```python
from build123d import *
from build123d.topology import SkipClean

# Parameters (mm, degrees)
SKETCH1_3_W             = 80
SKETCH1_3_H             = 80
SKETCH1_3_R             = 15
SKETCH1_3_R_2           = 2.5
BOSS_EXTRUDE3_DEPTH     = 5
BOSS_EXTRUDE4_START     = 5
SKETCH1_W               = 80
SKETCH1_H               = 80
SKETCH1_R               = 2.5
SKETCH1_R_2             = 25
BOSS_EXTRUDE4_DEPTH     = 5
CUT_EXTRUDE2_DEPTH      = 57.789083458
CUT_EXTRUDE2_DEPTH_BACK = 57.789083458
CUT_EXTRUDE3_DEPTH      = 57.789083608
CUT_EXTRUDE3_DEPTH_BACK = 57.789083608


with BuildPart() as part:
    # Sketch1_3 → Boss-Extrude3 (new body)
    with BuildSketch(Plane(origin=(0, 0, 0), x_dir=(1, 0, 0), z_dir=(0, 1, 0))):
        Rectangle(SKETCH1_3_W, SKETCH1_3_H)
        with Locations(Location((0, 0, 0), (0, 0, 270))):
            Circle(SKETCH1_3_R, mode=Mode.SUBTRACT)
        with Locations(Location((-32, 32, 0), (0, 0, 270))):
            Circle(SKETCH1_3_R_2, mode=Mode.SUBTRACT)
        with Locations(Location((-32, -32, 0), (0, 0, 270))):
            Circle(SKETCH1_3_R_2, mode=Mode.SUBTRACT)
        with Locations(Location((32, -32, 0), (0, 0, 270))):
            Circle(SKETCH1_3_R_2, mode=Mode.SUBTRACT)
        with Locations(Location((32, 32, 0), (0, 0, 270))):
            Circle(SKETCH1_3_R_2, mode=Mode.SUBTRACT)
    extrude(amount=-BOSS_EXTRUDE3_DEPTH)

    # Sketch1 → Boss-Extrude4 (add)
    with BuildSketch(Plane(origin=(0, 0, 0), x_dir=(1, 0, 0), z_dir=(0, 1, 0)).offset(BOSS_EXTRUDE4_START)):
        Rectangle(SKETCH1_W, SKETCH1_H)
        with Locations(Location((-32, -32, 0), (0, 0, 270))):
            Circle(SKETCH1_R, mode=Mode.SUBTRACT)
        with Locations(Location((32, -32, 0), (0, 0, 270))):
            Circle(SKETCH1_R, mode=Mode.SUBTRACT)
        with Locations(Location((0, 0, 0), (0, 0, 270))):
            Circle(SKETCH1_R_2, mode=Mode.SUBTRACT)
        with Locations(Location((-32, 32, 0), (0, 0, 270))):
            Circle(SKETCH1_R, mode=Mode.SUBTRACT)
        with Locations(Location((32, 32, 0), (0, 0, 270))):
            Circle(SKETCH1_R, mode=Mode.SUBTRACT)
    extrude(amount=-BOSS_EXTRUDE4_DEPTH)

    # Sketch3 → Cut-Extrude2 (cut, two sides: drawn at the far end of the back side and taken through both)
    with BuildSketch(Plane.XY.offset(-CUT_EXTRUDE2_DEPTH_BACK)):
        with BuildLine():
            Line((-40, 1.643191324), (-40, 5))
            Line((-40, 5), (0, 5))
            ThreePointArc((0, 5), (-20.070302467, 4.159325469), (-40, 1.643191324))
        make_face()
    extrude(amount=CUT_EXTRUDE2_DEPTH + CUT_EXTRUDE2_DEPTH_BACK, mode=Mode.SUBTRACT)

    # Sketch3_4 → Cut-Extrude3 (cut, two sides: drawn at the far end of the back side and taken through both)
    with SkipClean():  # the faces are left unmerged after this step: merging them gives an invalid solid
        with BuildSketch(Plane.XY.offset(-CUT_EXTRUDE3_DEPTH_BACK)):
            with BuildLine():
                Line((40, 5), (40, 1.643191324))
                ThreePointArc((40, 1.643191324), (20.070302467, 4.159325469), (0, 5))
                Line((0, 5), (40, 5))
            make_face()
        extrude(amount=CUT_EXTRUDE3_DEPTH + CUT_EXTRUDE3_DEPTH_BACK, mode=Mode.SUBTRACT)


solid = part.part
```
Verification items for the finished model (mm, model axes). A direction names the side the tool comes from. Coordinates: 2 decimals unless noted, no trailing zeros. Write each loop counter-clockwise with the first axis right and the second up, starting at its lowest first coordinate (ties: lowest second). Pieces come first, ordered by that corner, then holes. Notation, with made-up numbers: (-30, 41) - (15, 41) arc R20 ccw to (15, 47) - close; hole circle Ø10 at (-6, 87). An arc over 180 degrees is marked (long way). One line per question, with ' | ' between items. Start each with the question number.
1. Material ranges on line 1 along X through (y, z) = (-2.25, -32); line 2 along X through (y, z) = (0, -34); line 3 along Z through (x, y) = (0, 4), recorded low to high.
2. Section check B-B (z = 0). Enter the section's corners in (x, y), plus the area to 3 significant figures.
3. Section check C-C (y = -3.5). Enter the section's corners in (x, z), plus the area to 3 significant figures.
4. Access from +Z, -Z, +X, -X, +Y, -Y to the whole of each face (thin tool, end or side, straight path). Record for faces 1 (the cylindrical face through (7.509, 1.979, 23.846)), 2 (the flat face through (40, -2, 1)).
5. Draft check along X on faces 3 (the flat face through (-1, 0, 40)), 4 (the cylindrical face through (-29.52, -0.85, -32.33)), 5 (the flat face through (-40, -2, 1)). Enter one of: released by +X, released by -X, zero draft, split by the parting line, or undercut.
6. Section check A-A (x = 32). Enter the section's corners in (y, z).
7. Gauge pin test, flat ends, axial feed: P1, Ø8, axis at x = 11, z = 3.5, coming from the +Y side; P2, Ø6.5, axis at x = -32, z = 32, coming from the -Y side; P3, Ø8, axis at x = -32, z = -32, coming from the +Y side; P4, Ø6.5, axis at x = 32, z = -32, coming from the +Y side. Record the tip position at first contact, or that the pin passes through.
8. Section check D-D (x = 7). Enter the section's corners in (y, z), plus the area to 3 significant figures.
Computed values:
1) line 1: -40 to -34.5, -29.5 to 29.5, 34.5 to 40 | line 2: -40 to -33.5, -30.5 to 30.5, 33.5 to 40 | line 3: -40 to -25, 25 to 40
2) outline: (-40, -5) - (-15, -5) - (-15, 0) - (-25, 0) - (-25, 3.69) arc R240 ccw to (-40, 1.64) - close; (15, -5) - (40, -5) - (40, 1.64) arc R240 ccw to (25, 3.69) - (25, 0) - (15, 0) - close | area: 332 mm²
3) outline: (-40, -40) - (40, -40) - (40, 40) - (-40, 40) - close; hole circle Ø5 at (-32, -32); hole circle Ø5 at (-32, 32); hole circle Ø30 at (0, 0); hole circle Ø5 at (32, -32); hole circle Ø5 at (32, 32) | area: 5,610 mm²
4) face 1: +Y | face 2: +Z, -Z, +X, +Y, -Y
5) face 3: zero draft | face 4: undercut | face 5: released by -X
6) outline: (-5, -40) - (2.86, -40) - (2.86, -34.5) - (-5, -34.5) - close; (-5, -29.5) - (2.86, -29.5) - (2.86, 29.5) - (-5, 29.5) - close; (-5, 34.5) - (2.86, 34.5) - (2.86, 40) - (-5, 40) - close
7) P1: y = 0 | P2: y = -5 | P3: y = 3.36 | P4: y = 3.27
8) outline: (-5, -40) - (4.9, -40) - (4.9, -24) - (0, -24) - (0, -13.27) - (-5, -13.27) - close; (-5, 13.27) - (0, 13.27) - (0, 24) - (4.9, 24) - (4.9, 40) - (-5, 40) - close | area: 424 mm²
